Check sheet for the modelled part. Datum: model origin and axes. Units: mm. Give positions to 0.01 mm unless a question says otherwise; leave off trailing zeros. Order: outer loops, then holes, each group sorted by start corner. A loop starts at its lowest first (then second) coordinate and runs counter-clockwise, first axis right, second up. Notation, with made-up numbers: (-28.5, 76.5) -> (-21.5, 76.5) arc R24 ccw to (-21.5, 111.5) -> close; hole circle Ø9 at (21.5, -39.75). An arc over 180 degrees is marked (long way). One line per question, with ' | ' between items.
```python
from build123d import *

# Parameters (mm, degrees)
BOSS_EXTRUDE1_DEPTH = 2.2
SKETCH2_R           = 0.75
SKETCH2_R_2         = 2.5
CUT_EXTRUDE1_DEPTH  = 10


with BuildPart() as part:
    # Sketch1 → Boss-Extrude1 (new body)
    with BuildSketch(Plane(origin=(0, 0, 0), x_dir=(1, 0, 0), z_dir=(0, 1, 0))):
        with BuildLine():
            Line((-54.5, 0), (-54.5, 81))
            Line((-54.5, 81), (-51, 81))
            Line((-51, 81), (-51, 116))
            ThreePointArc((-51, 116), (0, 136), (51, 116))
            Line((51, 116), (51, 81))
            Line((51, 81), (54.5, 81))
            Line((54.5, 81), (54.5, 0))
            Line((54.5, 0), (-54.5, 0))
        make_face()
    extrude(amount=BOSS_EXTRUDE1_DEPTH)

    # Sketch2 → Cut-Extrude1 (cut)
    with BuildSketch(Plane(origin=(0, 2.2, 0), x_dir=(1, 0, 0), z_dir=(0, 1, 0))):
        with Locations(Location((-49, 114.5, 0), (0, 0, 270))):
            Circle(SKETCH2_R)
        with Locations(Location((0, 100, 0), (0, 0, 270))):
            Circle(SKETCH2_R_2)
        with Locations(Location((0, 80, 0), (0, 0, 270))):
            Circle(SKETCH2_R_2)
    cut_extrude1 = extrude(amount=-CUT_EXTRUDE1_DEPTH, mode=Mode.SUBTRACT)

    # Mirror1: Cut-Extrude1 across plane
    add(cut_extrude1.mirror(Plane(origin=(0, 0, 0), x_dir=(0, 0, 1), z_dir=(1, 0, 0))), mode=Mode.SUBTRACT)


solid = part.part
```
Q1. Section check C-C (x = 40). Enter the section's corners in (y, z).
Result sheet:
outline: (0, -124.45) -> (2.2, -124.45) -> (2.2, 0) -> (0, 0) -> close
Q2. Section check D-D (z = -123). Enter the section's corners in (x, y), and give its area (3 significant figures).
Result sheet:
outline: (-42.21, 0) -> (42.21, 0) -> (42.21, 2.2) -> (-42.21, 2.2) -> close | area: 186 mm2
Q3. Section check B-B (y = 1.4). Enter the section's corners in (x, z) (3 decimals), and give its area (3 significant figures).
Result sheet:
outline: (-54.5, -81) -> (-51, -81) -> (-51, -116) arc R75.025 ccw to (51, -116) -> (51, -81) -> (54.5, -81) -> (54.5, 0) -> (-54.5, 0) -> close; hole circle Ø1.5 at (-49, -114.5); hole circle Ø5 at (0, -100); hole circle Ø5 at (0, -80); hole circle Ø1.5 at (49, -114.5) | area: 13,800 mm2
Q4. Depth check by flat-ended pin: pin 1 Ø4 at (x, z) = (0, -100) entering from +Y; pin 2 Ø2 at (x, z) = (-49, -114.5) entering from -Y; pin 3 Ø1 at (x, y) = (-1.5, 1.5) entering from -Z; pin 4 Ø1.1 at (x, y) = (52.5, 1) entering from -Z. Enter the tip coordinate at first touch or a pass-through.
Result sheet:
pin 1: passes through | pin 2: stops at y = 0 | pin 3: stops at z = -135.99 | pin 4: stops at z = -81
Q5. Thickness scan on line 1 (X direction, y = 1.3, z = -80); line 2 (X direction, y = 1.1, z = -100); line 3 (Z direction, x = -49, y = 1.35). Record the ranges inside material, lowest first.
Result sheet:
line 1: x = -54.5 to -2.5, 2.5 to 54.5 | line 2: x = -51 to -2.5, 2.5 to 51 | line 3: z = -117.79 to -115.25, -113.75 to 0
Q6. Section check A-A (z = -100). Enter the section's corners in (x, y), and give its area (3 significant figures).
Result sheet:
outline: (-51, 0) -> (-2.5, 0) -> (-2.5, 2.2) -> (-51, 2.2) -> close; (2.5, 0) -> (51, 0) -> (51, 2.2) -> (2.5, 2.2) -> close | area: 213 mm2
Q7. Mould release check, pull along X, two halves, no side actions. Record for faces 1 (the face through (0.1, 1.1, -82.5)), 2 (the face through (1, 2.2, -69)), 3 (the face through (-0.785, 1.085, -135.996)): pulls with the +X half, pulls with the -X half, needs draft (parallel to the pull), parting line crosses it, or undercut.
Result sheet:
face 1: undercut | face 2: needs draft | face 3: parting line crosses it
